from build123d import *

# Parameters (mm, degrees)
SKETCH1_W           = 50
SKETCH1_H           = 50
SKETCH1_R           = 2
BOSS_EXTRUDE1_DEPTH = 1
SKETCH2_R           = 2
BOSS_EXTRUDE2_DEPTH = 70
CUT_EXTRUDE1_START  = -9.5
SKETCH7_R           = 2
CUT_EXTRUDE1_DEPTH  = 9.5
CUT_EXTRUDE2_START  = -10
SKETCH9_R           = 2
CUT_EXTRUDE2_DEPTH  = 10


with BuildPart() as part:
    # Sketch1 → Boss-Extrude1 (new body)
    with BuildSketch(Plane(origin=(0, 0, 0), x_dir=(1, 0, 0), z_dir=(0, 1, 0))):
        with Locations((25, 25)):
            Rectangle(SKETCH1_W, SKETCH1_H)
        with Locations(Location((25, 25, 0), (0, 0, 270))):
            Circle(SKETCH1_R, mode=Mode.SUBTRACT)
    extrude(amount=BOSS_EXTRUDE1_DEPTH)

    # Sketch2 → Boss-Extrude2 (add)
    with BuildSketch(Plane(origin=(0, 1, 0), x_dir=(1, 0, 0), z_dir=(0, 1, 0))):
        with Locations(Location((5, 45, 0), (0, 0, 90))):
            Circle(SKETCH2_R)
        with Locations(Location((45, 45, 0), (0, 0, 90))):
            Circle(SKETCH2_R)
    extrude(amount=BOSS_EXTRUDE2_DEPTH)

    # Sketch7 → Cut-Extrude1 (cut)
    with BuildSketch(Plane(origin=(0, 71, 0), x_dir=(1, 0, 0), z_dir=(0, 1, 0)).offset(CUT_EXTRUDE1_START)):
        with Locations(Location((5, 45, 0), (0, 0, 90))):
            Circle(SKETCH7_R)
        with Locations(Location((45, 45, 0), (0, 0, 90))):
            Circle(SKETCH7_R)
    extrude(amount=CUT_EXTRUDE1_DEPTH, mode=Mode.SUBTRACT)

    # Sketch9 → Cut-Extrude2 (cut)
    with BuildSketch(Plane(origin=(0, 61.5, 0), x_dir=(1, 0, 0), z_dir=(0, 1, 0)).offset(CUT_EXTRUDE2_START)):
        with Locations(Location((5, 45, 0), (0, 0, 90))):
            Circle(SKETCH9_R)
        with Locations(Location((45, 45, 0), (0, 0, 90))):
            Circle(SKETCH9_R)
    extrude(amount=CUT_EXTRUDE2_DEPTH, mode=Mode.SUBTRACT)


solid = part.part
The model under review builds one solid part; all positions refer to its coordinate system, in mm. A direction names the side the tool comes from. Round coordinates to 2 decimals unless told otherwise and drop trailing zeros. Order: outer loops, then holes, each group sorted by start corner. A loop starts at its lowest first (then second) coordinate and runs counter-clockwise, first axis right, second up. Notation, with made-up numbers: (-23, 85) - (16, 85) arc R11 ccw to (16, 97) - close; hole circle Ø3 at (17, -7.5). An arc over 180 degrees is marked (long way). Use one line per item in the form item = value.
Q1. To check wall thickness, follow line 1 (X direction, y = 0.75, z = -25); line 2 (X direction, y = 3, z = -45); line 3 (Y direction, x = 18.5, z = -23). State the ranges of each line that lie inside material, in increasing order.
Response values:
line_1 = 0 to 23, 27 to 50
line_2 = 3 to 7, 43 to 47
line_3 = 0 to 1
Q2. Mouldability with a two-part tool opening along Z and no side actions: class faces 1 (the flat face through (19, 0, -25)), 2 (the cylindrical face through (23.8, 0.5, -26.6)), 3 (the cylindrical face through (47, 26, -45)) as pulls with the +Z half, pulls with the -Z half, needs draft (parallel to the pull), parting line crosses it, or undercut.
Response values:
face_1 = needs draft
face_2 = undercut
face_3 = parting line crosses it
Q3. Clearance check with flat-ended pins moving along their axes: P1, Ø12, axis at x = 12, z = -15, coming from the -Y side; P2, Ø3, axis at x = 8, y = 31, coming from the +Z side; P3, Ø6, axis at x = 38.5, z = -12, coming from the +Y side. State where each tip first meets the part, or that it passes through.
Response values:
P1 = 0
P2 = -43.68
P3 = 1
Q4. Add section A-A on x = 25. Give the boundary of the cut face in (y, z).
Response values:
outline = (0, -50) - (1, -50) - (1, -27) - (0, -27) - close; (0, -23) - (1, -23) - (1, 0) - (0, 0) - close
Q5. Add section B-B on z = -25. Give the boundary of the cut face in (x, y), then the cut area to 3 significant figures.
Response values:
outline = (0, 0) - (23, 0) - (23, 1) - (0, 1) - close; (27, 0) - (50, 0) - (50, 1) - (27, 1) - close
area = 46.0 mm^2
Q6. Add section C-C on x = 5. Give the boundary of the cut face in (y, z).
Response values:
outline = (0, -50) - (1, -50) - (1, -47) - (51.5, -47) - (51.5, -43) - (1, -43) - (1, 0) - (0, 0) - close
Q7. Tool access review of faces 4 (the cylindrical face through (5, 26, -43)), 5 (the flat face through (45, 51.5, -45)): name each direction out of +Z, -Z, +X, -X, +Y, -Y from which nothing blocks a thin tool from reaching the whole face with its end or side.
Response values:
face_4 = +Y
face_5 = +Z, -Z, +X, -X, +Y
Q8. Add section D-D on y = 8.5. Give the boundary of the cut face in (x, z), then the cut area to 3 significant figures.
Response values:
outline = circle Ø4 at (5, -45); circle Ø4 at (45, -45)
area = 25.1 mm^2
